Work out the finished part from the listing and answer in its coordinate system (mm). A direction names the side the tool comes from. Coordinates: 2 decimals unless noted, no trailing zeros. Write each loop counter-clockwise with the first axis right and the second up, starting at its lowest first coordinate (ties: lowest second). Pieces come first, ordered by that corner, then holes. Notation, with made-up numbers: (35.25, 41) - (59.25, 41) arc R24 ccw to (59.25, 52) - close; hole circle Ø8 at (-4.75, 7.25). An arc over 180 degrees is marked (long way). Use one line per item in the form item = value. Start each with the question number.
Item 1: Consider probe 1 along Y at (x, z) = (3, 1.05); probe 2 along Y at (x, z) = (-2.75, 0.3). Determine where each line is inside the solid, lowest interval first.
Item 2: A cutting plane is placed at D-D (y = -1.3). Write down the section's boundary in (x, z).
Item 3: For faces 4 (the flat face through (4, 2, 1)), 5 (the flat face through (4, 0, 1)), determine the directions among +Z, -Z, +X, -X, +Y, -Y from which every point of the face is accessible in a straight line to the end or side of a thin tool.
Item 4: Determine the mould class of faces 1 (the flat face through (-16.394, -1.909, 0.769)), 2 (the flat face through (9.89, 0.99, 0.75)), 3 (the flat face through (-1.94, 0.13, 1.397)) for opening direction X: released by +X, released by -X, zero draft, split by the parting line, or undercut.
Item 5: A cutting plane is placed at B-B (y = 0.6). Write down the section's boundary in (x, z).
Item 6: Given pin 1 (1 mm diameter, centred on x = 2, y = -1, fed in from -Z); pin 2 (0.6 mm diameter, centred on x = 4.5, z = 0.5, fed in from -Y), each flat-ended and moving along its own axis, determine where each tip first touches the part or whether it passes through.
Item 7: A cutting plane is placed at A-A (z = 0.5). Write down the section's boundary in (x, y), then the cut area to 3 significant figures.
Item 8: A cutting plane is placed at C-C (x = -3.5). Write down the section's boundary in (y, z), then the cut area to 3 significant figures.
from build123d import *

# Parameters (mm, degrees)
BOSS_EXTRUDE2_DEPTH = 2
BOSS_EXTRUDE4_DEPTH = 1.274755


with BuildPart() as part:
    # Sketch1 → Boss-Extrude2 (new body)
    with BuildSketch(Plane(origin=(0, 0, 0), x_dir=(1, 0, 0), z_dir=(0, 1, 0))):
        Polygon((-1.878719766, -1.397030535), (-1.878719766, -0.122275657), (6.747505842, -0.122275657), (13.121280234, -1.397030535), align=None)
    extrude(amount=BOSS_EXTRUDE2_DEPTH)

    # Sketch4 → Boss-Extrude4 (add)
    with BuildSketch(Plane.XY.offset(1.397030535)):
        Polygon((-1.878719766, 2), (-16.587429902, -0.941742026), (-16.195197632, -2.902903377), (-1.486487496, 0.038838649), align=None)
    extrude(amount=-BOSS_EXTRUDE4_DEPTH)


solid = part.part
Answer:
q1.probe_1 = 0 to 2
q1.probe_2 = -0.21 to 1.83
q2.outline = (-16.52, 0.12) - (-8.18, 0.12) - (-8.18, 1.4) - (-16.52, 1.4) - close
q3.face_4 = +Z, -Z, +X, -X, +Y
q3.face_5 = +Z, -Z, +X, -Y
q4.face_1 = released by -X
q4.face_2 = released by +X
q4.face_3 = zero draft
q5.outline = (-8.88, 0.12) - (6.75, 0.12) - (13.12, 1.4) - (-8.88, 1.4) - close
q6.pin_1 = through
q6.pin_2 = 0
q7.outline = (-16.59, -0.94) - (-16.2, -2.9) - (-1.68, 0) - (8.64, 0) - (8.64, 2) - (-1.88, 2) - close
q7.area = 50.6 mm²
q8.outline = (-0.36, 0.12) - (1.68, 0.12) - (1.68, 1.4) - (-0.36, 1.4) - close
q8.area = 2.60 mm²
